Model file for the job. Use its own axes, mm. A direction names the side the tool comes from. Round coordinates to 2 decimals unless told otherwise and drop trailing zeros. Order: outer loops, then holes, each group sorted by start corner. A loop starts at its lowest first (then second) coordinate and runs counter-clockwise, first axis right, second up. Notation, with made-up numbers: (-39.5, 54.5) -> (-28.5, 54.5) arc R17 cw to (-28.5, 59.5) -> close; hole circle Ø3 at (8.25, 60). An arc over 180 degrees is marked (long way). Answer as CSV lines item,"result".
```python
from build123d import *

# Parameters (mm, degrees)
SKETCH_1_W           = 140
SKETCH_1_H           = 175
EXTRUDE_1_DEPTH      = 150
SKETCH_2_W           = 110
SKETCH_2_H           = 145
CUT_EXTRUDE_1_DEPTH  = 150
SKETCH_3_W           = 115
SKETCH_3_H           = 145
CUT_EXTRUDE_2_DEPTH  = 150
SKETCH_4_W           = 110
SKETCH_4_H           = 135
CUT_EXTRUDE_3_DEPTH  = 150
SKETCH_5_W           = 20
SKETCH_5_H           = 40
CUT_EXTRUDE_4_DEPTH  = 150
SKETCH_6_W           = 20
SKETCH_6_H           = 115
CUT_EXTRUDE_5_DEPTH  = 150
EXTRUDE_2_DEPTH      = 30
CUT_EXTRUDE_6_DEPTH  = 30
SKETCH_9_W           = 30
SKETCH_9_H           = 30
CUT_EXTRUDE_7_DEPTH  = 15
SKETCH_10_W          = 20
SKETCH_10_H          = 60
CUT_EXTRUDE_8_DEPTH  = 20
EXTRUDE_3_DEPTH      = 5
EXTRUDE_4_DEPTH      = 5
EXTRUDE_1_2_DEPTH    = 10
EXTRUDE_2_2_DEPTH    = 10
FILLET_1_R           = 10
CUT_EXTRUDE_9_DEPTH  = 52
CUT_EXTRUDE_10_DEPTH = 52
FILLET_2_R           = 20
FILLET_3_R           = 10


with BuildPart() as part:
    # 草图1 → Extrude 1 (new body)
    with BuildSketch(Plane.XY):
        Rectangle(SKETCH_1_W, SKETCH_1_H)
    extrude(amount=EXTRUDE_1_DEPTH)

    # 草图2 → 切除-拉伸1 (cut)
    with BuildSketch(Plane.XY.offset(150)):
        with Locations((-15, -15)):
            Rectangle(SKETCH_2_W, SKETCH_2_H)
    extrude(amount=-CUT_EXTRUDE_1_DEPTH, mode=Mode.SUBTRACT)

    # 草图3 → 切除-拉伸2 (cut)
    with BuildSketch(Plane.ZY.offset(-40)):
        with Locations((57.5, -15)):
            Rectangle(SKETCH_3_W, SKETCH_3_H)
    extrude(amount=-CUT_EXTRUDE_2_DEPTH, mode=Mode.SUBTRACT)

    # 草图4 → 切除-拉伸3 (cut)
    with BuildSketch(Plane.XZ.offset(-57.5)):
        with Locations((15, 67.5)):
            Rectangle(SKETCH_4_W, SKETCH_4_H)
    extrude(amount=-CUT_EXTRUDE_3_DEPTH, mode=Mode.SUBTRACT)

    # 草图5 → 切除-拉伸4 (cut)
    with BuildSketch(Plane.XZ.offset(87.5)):
        with Locations((55, 115)):
            Rectangle(SKETCH_5_W, SKETCH_5_H)
    extrude(amount=-CUT_EXTRUDE_4_DEPTH, mode=Mode.SUBTRACT)

    # 草图6 → 切除-拉伸5 (cut)
    with BuildSketch(Plane.ZY.offset(-40)):
        with Locations((125, 0)):
            Rectangle(SKETCH_6_W, SKETCH_6_H)
    extrude(amount=-CUT_EXTRUDE_5_DEPTH, mode=Mode.SUBTRACT)

    # 草图7 → Extrude 2 (add)
    with BuildSketch(Plane.XY.offset(150)):
        Polygon((-70, 57.5), (40, 57.5), (40, -87.5), (70, -87.5), (70, 87.5), (-70, 87.5), align=None)
    extrude(amount=EXTRUDE_2_DEPTH)

    # 草图8 → 切除-拉伸6 (cut)
    with BuildSketch(Plane(origin=(0, 0, 135), x_dir=(-1, 0, 0), z_dir=(0, 0, -1))):
        Polygon((-65, -57.5), (-45, -57.5), (-40, -57.5), (-40, 57.5), (40, 57.5), (40, 87.5), (-70, 87.5), (-70, -57.5), align=None)
    extrude(amount=-CUT_EXTRUDE_6_DEPTH, mode=Mode.SUBTRACT)

    # 草图9 → 切除-拉伸7 (cut)
    with BuildSketch(Plane(origin=(0, 0, 0), x_dir=(-1, 0, 0), z_dir=(0, 0, -1))):
        with Locations((55, 72.5)):
            Rectangle(SKETCH_9_W, SKETCH_9_H)
    extrude(amount=-CUT_EXTRUDE_7_DEPTH, mode=Mode.SUBTRACT)

    # 草图10 → 切除-拉伸8 (cut)
    with BuildSketch(Plane(origin=(0, 0, 15), x_dir=(-1, 0, 0), z_dir=(0, 0, -1))):
        with Locations((55, 87.5)):
            Rectangle(SKETCH_10_W, SKETCH_10_H)
    extrude(amount=-CUT_EXTRUDE_8_DEPTH, mode=Mode.SUBTRACT)

    # 草图11 → 凸台-拉伸3 (add)
    with BuildSketch(Plane(origin=(0, 87.5, 0), x_dir=(1, 0, 0), z_dir=(0, 1, 0))):
        Polygon((-40, -35), (70, -165), (-40, -165), align=None)
    extrude(amount=-EXTRUDE_3_DEPTH)

    # 草图12 → 凸台-拉伸4 (add)
    with BuildSketch(Plane.XY.offset(180)):
        Polygon((-70, 57.5), (40, -87.5), (40, 57.5), align=None)
    extrude(amount=-EXTRUDE_4_DEPTH)

    # 草图13 → Extrude 1 2 (add)
    with BuildSketch(Plane(origin=(0, 0, 175), x_dir=(-1, 0, 0), z_dir=(0, 0, -1))):
        Polygon((70, 57.5), (-40, -87.5), (-47.966912709, -81.456135186), (62.033087291, 63.543864814), align=None)
    extrude(amount=EXTRUDE_1_2_DEPTH)

    # 草图14 → Extrude 2 2 (add)
    with BuildSketch(Plane.XZ.offset(-82.5)):
        Polygon((-40, 35), (70, 165), (62.366137146, 171.459422415), (-47.633862854, 41.459422415), align=None)
    extrude(amount=EXTRUDE_2_2_DEPTH)

    # 圆角1
    fillet_1_edges = [part.edges().sort_by_distance(p)[0] for p in [
        (8.450236013, 82.5, 107.740630166),
        (-8.724043199, -6.727147853, 175),
    ]]
    fillet(fillet_1_edges, radius=FILLET_1_R - 0.0001)  # a hair under: the kernel refuses the full size

    # 草图15 → 切除-拉伸9 (cut)
    with BuildSketch(Plane(origin=(0, 0, 175), x_dir=(-1, 0, 0), z_dir=(0, 0, -1))):
        Polygon((-40, 57.5), (-40, -54.408591412), (44.896172796, 57.5), align=None)
    extrude(amount=-CUT_EXTRUDE_9_DEPTH, mode=Mode.SUBTRACT)

    # 草图16 → 切除-拉伸10 (cut)
    with BuildSketch(Plane.XZ.offset(-82.5)):
        Polygon((-40, 165), (-40, 65.962520665), (43.800944052, 165), align=None)
    extrude(amount=-CUT_EXTRUDE_10_DEPTH, mode=Mode.SUBTRACT)

    # 圆角2
    fillet_2_edges = [part.edges().sort_by_distance(p)[0] for p in [
        (40, 57.5, 172.5),
        (-40, 72.5, 165),
    ]]
    fillet(fillet_2_edges, radius=FILLET_2_R)

    # 圆角3
    fillet_3_edges = [part.edges().sort_by_distance(p)[0] for p in [
        (55, -57.5, 165),
    ]]
    fillet(fillet_3_edges, radius=FILLET_3_R)


solid = part.part
```
Q1. Tool access for faces 1 (the cylindrical face through (-7.134, -4.105, 171.993)), 2 (the flat face through (14.23, 80.1, 99.09)), 3 (the flat face through (45, -73, 125)), 4 (the flat face through (46, 36, 165)): list every direction of +Z, -Z, +X, -X, +Y, -Y with a clear straight run to the whole face (end or side of a thin tool).
Checks:
face 1,"-Z"
face 2,"-Z, +X, +Y"
face 3,"-Z, +Y, -Y"
face 4,"none"
Q2. Saw through at A-A (y = 76.5). Write the cut outline in (x, z), plus the area to 3 significant figures.
Checks:
outline,"(-70, 15) -> (-65, 15) -> (-65, 35) -> (-45, 35) -> (-45, 15) -> (-40, 15) -> (-40, 35) -> (70, 165) -> (70, 180) -> (-70, 180) -> close; hole (-40, 51.77) -> (55.81, 165) -> (-20, 165) arc R20 ccw to (-40, 145) -> close"
area,"8,010 mm²"
Q3. Saw through at D-D (z = 43). Write the cut outline in (x, y), plus the area to 3 significant figures.
Checks:
outline,"(-70, 57.5) -> (-40, 57.5) -> (-40, 72.5) -> (-33.23, 72.5) -> (-33.23, 87.5) -> (-70, 87.5) -> close"
area,"1,000 mm²"
Q4. Mould opens along X. For faces 5 (the cylindrical face through (5.476, 79.648, 108.881)), 6 (the flat face through (70, -40, 169)), 7 (the flat face through (11, 72.5, 100)) say: +X half, -X half, draft (parallel to the pull), parting line (faces both ways), or undercut.
Checks:
face 5,"undercut"
face 6,"+X half"
face 7,"draft"
Q5. Saw through at B-B (z = 140). State how many separate pieces and enclosed holes the cut face has, plus the area to 3 significant figures.
Checks:
separate pieces,"3"
enclosed holes,"0"
area,"2,090 mm²"
Q6. Wall check: L1, parallel to Z at x = -50, y = 71.5; L2, parallel to Y at x = -49, z = 124.5; L3, parallel to X at y = -77, z = 151. Give the ranges that are in metal, low to high. Write a range as [from, to].
Checks:
L1,"[35, 180]"
L2,"[57.5, 87.5]"
L3,"[40, 70]"
Q7. Flat gauge pins, fed straight in: pin 1 (2.5 mm diameter, centred on x = 67.5, y = -72.5, fed in from -Z); pin 2 (22 mm diameter, centred on y = 70, z = 20.5, fed in from +X); pin 3 (6 mm diameter, centred on x = 51.5, y = -72, fed in from -Z). Where does each tip first touch, or does it go through?
Checks:
pin 1,"z = 115"
pin 2,"x = -40"
pin 3,"z = 135"
